Autodesk Inventor part; units mm, degrees
ref_plane "YZ Plane" through (0, 0, 0) normal (1, 0, 0) x (0, 1, 0)
ref_plane "XZ Plane" through (0, 0, 0) normal (0, 1, 0) x (-1, 0, 0)
ref_plane "XY Plane" through (0, 0, 0) normal (0, 0, 1) x (1, 0, 0)
sketch "Sketch1" plane through (0, 0, 0) normal (0, 0, 1) x (1, 0, 0)
  line L0 (6.35, 28.575) -> (25.4, 28.575)
  line L1 (6.35, 31.75) -> (25.4, 31.75)
  line L2 (25.4, 0) -> (6.35, 0)
  arc A0 (0, 6.35) -> (6.35, 0) centre (6.35, 6.35) ccw
  line L3 (0, 6.35) -> (0, 25.4)
  arc A1 (6.35, 31.75) -> (0, 25.4) centre (6.35, 25.4) ccw
  line L4 (6.35, 31.75) -> (25.4, 31.75)
  line L5 (25.4, 28.575) -> (6.35, 28.575)
  arc A2 (6.35, 28.575) -> (3.175, 25.4) centre (6.35, 25.4) ccw
  line L6 (3.175, 25.4) -> (3.175, 6.35)
  arc A3 (3.175, 6.35) -> (6.35, 3.175) centre (6.35, 6.35) ccw
  line L7 (6.35, 3.175) -> (25.4, 3.175)
  line L8 (28.575, 3.175) -> (28.575, 0)
  line L9 (25.4, 31.75) -> (28.575, 31.75)
  line L10 (28.575, 28.575) -> (25.4, 28.575)
  line L11 (28.575, 31.75) -> (28.575, 28.575)
  line L12 (28.575, 0) -> (25.4, 0)
  line L13 (28.575, 3.175) -> (28.575, 0)
  line L14 (25.4, 3.175) -> (28.575, 3.175)
  point P0 (0, 0)
extrude "Extrusion1" add sketch "Sketch1" against normal blind 762
chamfer "Chamfer1" distance 3.175 angle 45 4 edges at (28.575, 30.1625, 0) (28.575, 1.5875, 0) (28.575, 30.1625, -762) (28.575, 1.5875, -762)
sketch "Sketch2" plane through (6.35, 31.75, 0) normal (0, 1, 0) x (1, 0, 0)
  line L0 (19.05, 0) -> (0, 0)
  line L1 (22.225, 3.175) -> (22.225, 758.825)
  point P0 (-6.35, 0)
  point P1 (9.525, 12.7)
  dimension "d5" = 12.7
  dimension "d6" = 12.7
hole "Hole1" at (15.875, 31.75, -12.7) direction (0, -1, 0) diameter 6.7056 end through all
pattern_linear "Rectangular Pattern1" count 30 spacing 25.4 along (0, 0, -1) of "Hole1"
sketch "Sketch3" plane through (0, 6.35, 0) normal (-1, 0, 0) x (0, 0, 1)
  line L0 (-0.2722, 19.0092) -> (-759.0056, 19.0092)
  line L1 (-759.0056, 19.0092) -> (-759.0056, 0.0408)
  line L2 (-0.2722, 0.0408) -> (-759.0056, 0.0408)
  line L3 (-0.2722, 0.0408) -> (-0.2722, 19.0092)
  circle A0 centre (-698.5852, 9.525) radius 4.78
  circle A1 centre (-111.2243, 9.525) radius 4.78
  circle A2 centre (-188.7416, 9.525) radius 3.6672
  circle A3 centre (-277.2605, 9.525) radius 3.6672
  circle A4 centre (-481.9921, 9.525) radius 3.6672
  circle A5 centre (-570.511, 9.525) radius 3.6672
  circle A6 centre (-469.3591, 9.525) radius 3.6672
  circle A7 centre (-583.1692, 9.525) radius 3.6672
  circle A8 centre (-289.9187, 9.525) radius 3.6672
  circle A9 centre (-176.1087, 9.525) radius 3.6672
  circle A10 centre (-551.6311, 9.525) radius 4.78
  circle A11 centre (-526.34, 9.525) radius 4.78
  circle A12 centre (-501.0489, 9.525) radius 4.78
  circle A13 centre (-258.2289, 9.525) radius 4.78
  circle A14 centre (-232.9378, 9.525) radius 4.78
  circle A15 centre (-207.6467, 9.525) radius 4.78
  circle A16 centre (-607.2589, 9.525) radius 1.5807
  circle A17 centre (-152.0189, 9.525) radius 1.5807
  circle A18 centre (-379.6389, 5.9842) radius 4.78
  circle A19 centre (-85.9332, 9.525) radius 4.78
  circle A20 centre (-673.294, 9.525) radius 4.78
  circle A21 centre (-648.0029, 9.525) radius 4.78
  circle A22 centre (-63.5, 9.525) radius 4.8006
  point P0 (0, -6.35)
  point P1 (-759.0056, -6.2819)
  dimension "d21" = 9.6012
extrude "Extrusion2" [suppressed]
sketch "Sketch4" plane through (6.35, 31.75, 0) normal (0, 1, 0) x (1, 0, 0)
  line L0 (-18.2452, 26.2664) -> (88.0083, 26.2664)
  line L1 (88.0083, 26.2664) -> (88.0083, 1027.7541)
  line L2 (88.0083, 1027.7541) -> (-18.2452, 1027.7541)
  line L3 (-18.2452, 1027.7541) -> (-18.2452, 26.2664)
  point P0 (-6.35, 0)
extrude "Extrusion3" cut sketch "Sketch4" against normal blind 50.8
sketch "Sketch5" plane through (0, 6.35, 0) normal (-1, 0, 0) x (0, 0, 1)
  circle A0 centre (-63.5, 9.525) radius 4.8006
  dimension "d23" = 9.6012
extrude "Extrusion4" cut sketch "Sketch5" against normal through all
fillet "Fillet1" radius 3.175 2 edges at (28.575, 30.1625, -26.2664) (28.575, 1.5875, -26.2664)
properties part number "niblet" material "Aluminum 6061"
Part model, mm, in its own coordinate system. A direction names the side the tool comes from. Round coordinates to 2 decimals unless told otherwise and drop trailing zeros. Loops run counter-clockwise (first coordinate to the right, second up) from the corner with the lowest first, then second, coordinate; pieces in that order, holes last.
Item 1: Cut at C-C, the plane z = -22.5. Give the cut face in (x, y) (3 decimals), then the cut area to 3 significant figures.
Item 2: Cut at B-B, the plane x = 24. Give the cut face in (y, z) (3 decimals).
Item 3: Cut at A-A, the plane z = -12.7. Give the cut face in (x, y) (3 decimals).
Item 4: Drop flat-ended pins along their axis: P1, Ø11, axis at x = 19, z = -13, coming from the -Y side; P2, Ø10, axis at y = 21.5, z = -18, coming from the +X side; P3, Ø15, axis at y = 12.5, z = -11, coming from the +X side; P4, Ø4, axis at y = 15, z = -16, coming from the +X side (3 decimals). Give the stop position or say it passes through.
Item 5: Mould opens along X. For faces 1 (the face through (1.81, 1.91, -12.95)), 2 (the face through (17.915, 30.14, -15.361)), 3 (the face through (17.915, 1.565, -15.361)), 4 (the face through (28.575, 2, -13)) say: +X half, -X half, draft (parallel to the pull), parting line (faces both ways), or undercut.
Item 6: Cut at D-D, the plane y = 12. Give the cut face in (x, z) (3 decimals).
Item 7: 3-axis set-ups, long thin cutter, end or side, ignore diameter. For faces 5 (the face through (27.67, 30.18, -25.31)), 6 (the face through (20, 28.575, -13)): which of +Z, -Z, +X, -X, +Y, -Y reach the whole face in a straight line?
Item 8: Drill centre lines: line 1 (Y direction, x = 19.75, z = -10.75) (3 decimals); line 2 (X direction, y = 10, z = -23.75) (3 decimals); line 3 (X direction, y = 30.25, z = -12.7) (3 decimals). Where is each one in solid material? Low to high.
A:
1. outline: (0, 6.35) arc R6.35 ccw to (6.35, 0) - (28.575, 0) - (28.575, 3.175) - (6.35, 3.175) arc R3.175 cw to (3.175, 6.35) - (3.175, 25.4) arc R3.175 cw to (6.35, 28.575) - (28.575, 28.575) - (28.575, 31.75) - (6.35, 31.75) arc R6.35 ccw to (0, 25.4) - close
1. area: 249 mm2
2. outline: (0, -26.266) - (3.175, -26.266) - (3.175, 0) - (0, 0) - close; (28.575, -26.266) - (31.75, -26.266) - (31.75, 0) - (28.575, 0) - close
3. outline: (0, 6.35) arc R6.35 ccw to (6.35, 0) - (12.522, 0) - (12.522, 3.175) - (6.35, 3.175) arc R3.175 cw to (3.175, 6.35) - (3.175, 25.4) arc R3.175 cw to (6.35, 28.575) - (12.522, 28.575) - (12.522, 31.75) - (6.35, 31.75) arc R6.35 ccw to (0, 25.4) - close; (19.228, 0) - (28.575, 0) - (28.575, 3.175) - (19.228, 3.175) - close; (19.228, 28.575) - (28.575, 28.575) - (28.575, 31.75) - (19.228, 31.75) - close
4. P1: stops at y = 0
4. P2: stops at x = 3.37
4. P3: stops at x = 3.48
4. P4: stops at x = 3.175
5. face 1: -X half
5. face 2: undercut
5. face 3: undercut
5. face 4: +X half
6. outline: (0, -26.266) - (3.175, -26.266) - (3.175, 0) - (0, 0) - close
7. face 5: -Z, +X, +Y, -Y
7. face 6: +Z, -Z, +X
8. line 1: y = 0 to 3.175, 28.575 to 31.75
8. line 2: x = 0 to 3.175
8. line 3: x = 2.251 to 12.522, 19.228 to 28.575
